The model under review builds one solid part; all positions refer to its coordinate system, in mm. A direction names the side the tool comes from. Coordinates: 2 decimals unless noted, no trailing zeros. Order: outer loops, then holes, each group sorted by start corner. A loop starts at its lowest first (then second) coordinate and runs counter-clockwise, first axis right, second up.
from build123d import *

# Parameters (mm, degrees)
BOSS_EXTRUDE1_DEPTH      = 3
BOSS_EXTRUDE1_DEPTH_BACK = 6
SKETCH1_R                = 10
SKETCH4_R                = 1.6
HOLE_DEPTH               = 19.539009706
HOLECIR_COUNT            = 5
FILLET3_R                = 2


with BuildPart() as part:
    # Sketch1 → Boss-Extrude1 (new, two sides: drawn at the far end of the back side and taken through both)
    with BuildSketch(Plane(origin=(0, 0, 0), x_dir=(1, 0, 0), z_dir=(0, 1, 0)).offset(-BOSS_EXTRUDE1_DEPTH_BACK)):
        with Locations(Location((0, 0, 0), (0, 0, 270))):
            Circle(SKETCH1_R)
    extrude(amount=BOSS_EXTRUDE1_DEPTH + BOSS_EXTRUDE1_DEPTH_BACK)

    # Sketch4 → hole (cut, through all)
    with BuildSketch(Plane(origin=(-3.352872105, -1.093066116, 1.887711608), x_dir=(-0.4486862613641547, -0.14627571033740308, -0.8816371449912632), z_dir=(0.8382180262940947, 0.2732665289126682, -0.47192790187872385))):
        with Locations(Location((0, 0, 0), (0, 0, 8.746528197))):
            Circle(SKETCH4_R)
    hole = extrude(amount=-HOLE_DEPTH, mode=Mode.SUBTRACT)

    # holecir: hole ×5 about axis
    holecir_axis = Axis((0, 0, 0), (0, 1, 0))
    for i in range(1, HOLECIR_COUNT):
        add(hole.rotate(holecir_axis, i * 360 / HOLECIR_COUNT), mode=Mode.SUBTRACT)

    # Fillet3
    fillet3_edges = [part.edges().sort_by_distance(p)[0] for p in [
        (0, 3, -10),
    ]]
    fillet(fillet3_edges, radius=FILLET3_R)


solid = part.part
(1) Consider section B-B (x = -3.5). Give the number of separate pieces and of enclosed holes in the cut face, then the cut area to 3 significant figures.
(2) Insertion check: pin 1 Ø1.5 at (x, y) = (1, -0.5) entering from -Z; pin 2 Ø5 at (y, z) = (-3.5, 6.5) entering from +X. Each pin has a flat end and moves straight along its axis. Give the tip position at first contact, or say it passes through.
(3) Tool access review of faces 4 (the face through (0, 3, 0)), 5 (the face through (1.59, -1.07, -3.51)): name each direction out of +Z, -Z, +X, -X, +Y, -Y from which nothing blocks a thin tool from reaching the whole face with its end or side.
(4) Consider section A-A (y = 2.75). Give the boundary of the cut face in (x, z), then the cut area to 3 significant figures.
(5) Wall thickness on line 1 (Z direction, x = -3.75, y = 0); line 2 (Z direction, x = -7.75, y = -3.5); line 3 (X direction, y = -3, z = 7.5): over which ranges is each line inside the solid? List them lowest first.
(6) The part is to be moulded in two halves that separate along Z. For faces 1 (the face through (0, -6, 0)), 2 (the face through (-3.35, -1.07, 1.91)), 3 (the face through (6.76, -2.55, -7.37)), say which applies: +Z half, -Z half, draft (parallel to the pull), parting line (faces both ways), or undercut.
Findings:
1. separate pieces: 1
1. enclosed holes: 2
1. area: 151 mm2
2. pin 1: stops at z = -10
2. pin 2: stops at x = 9.17
3. face 4: +Z, -Z, +X, -X, +Y
3. face 5: none
4. outline: circle Ø17.94 at (0, 0)
4. area: 253 mm2
5. line 1: z = -9.27 to -4.13, -2.07 to 1.82, 3.16 to 9.27
5. line 2: z = -5.27 to 3.04, 6.01 to 6.32
5. line 3: x = -6.61 to 0.14, 2.97 to 6.61
6. face 1: draft
6. face 2: undercut
6. face 3: parting line
